Design review of the part shown in the three views and the two pictorial views. Dimensions are in mm from the part's minimum x, y and z. A direction names the side the tool comes from. Coordinates: 2 decimals unless noted, no trailing zeros. Loops run counter-clockwise (first coordinate to the right, second up) from the corner with the lowest first, then second, coordinate; pieces in that order, holes last. Notation, with made-up numbers: (-28.75, 60) -> (-12.75, 60) arc R30 cw to (-12.75, 83) -> close; hole circle Ø9 at (68.25, 35.25). An arc over 180 degrees is marked (long way). Answer in a Markdown table with one row per item.
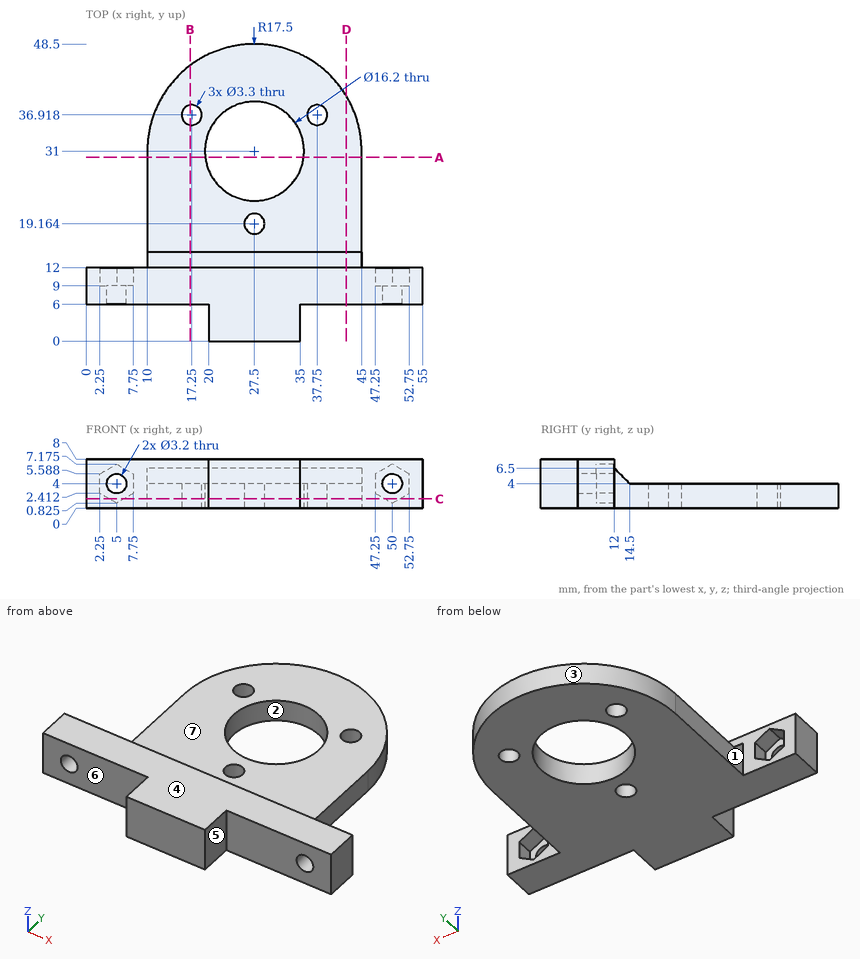
Item 1: For L1, parallel to Z at x = 50, y = 7; L2, parallel to X at y = 10.5, z = 2.25; L3, parallel to Z at x = 14.5, y = 31.5, list the stretches that pass through material, from the lowest coordinate up.
Worked answers:
| item | result |
|---|---|
| L1 | 0 to 2.4, 5.6 to 8 |
| L2 | 0 to 2.53, 7.47 to 47.53, 52.47 to 55 |
| L3 | 0 to 4 |
Item 2: Take a section at A-A, the plane y = 30. State the section outline as (x, z) points.
Worked answers:
| item | result |
|---|---|
| outline | (10, 0) -> (19.46, 0) -> (19.46, 4) -> (10, 4) -> close; (35.54, 0) -> (45, 0) -> (45, 4) -> (35.54, 4) -> close |
Item 3: For the marked faces 4, 5, 6 and 7, list the 3-axis set-ups (+Z, -Z, +X, -X, +Y, -Y) from which the entire face can be reached by the end or side of a thin tool; tool diameter is ignored.
Worked answers:
| item | result |
|---|---|
| face 4 | +Z, +X, -X, +Y, -Y |
| face 5 | +Z, -Z, +X, -Y |
| face 6 | +Z, -Z, -X, -Y |
| face 7 | +Z, +X, -X, +Y |
Item 4: Take a section at D-D, the plane x = 42.5. State the section outline as (y, z) points, and give its area (3 significant figures).
Worked answers:
| item | result |
|---|---|
| outline | (6, 0) -> (40.01, 0) -> (40.01, 4) -> (14.5, 4) -> (12, 6.5) -> (12, 8) -> (6, 8) -> close |
| area | 163 mm² |
Item 5: Take a section at C-C, the plane z = 1.5. Count the separate pieces of the cut face and the enclosed holes in it, and give its area (3 significant figures).
Worked answers:
| item | result |
|---|---|
| separate pieces | 1 |
| enclosed holes | 4 |
| area | 1,320 mm² |
Item 6: The part is to be moulded in two halves that separate along X. For the marked faces 1, 2 and 3, say which applies: +X half, -X half, draft (parallel to the pull), parting line (faces both ways), or undercut.
Worked answers:
| item | result |
|---|---|
| face 1 | -X half |
| face 2 | undercut |
| face 3 | parting line |
Item 7: Insertion check: pin 1 (1.6 mm diameter, centred on x = 49.5, z = 3, fed in from +Y); pin 2 (4 mm diameter, centred on x = 45.5, z = 2.5, fed in from -Y); pin 3 (1 mm diameter, centred on y = 32, z = 1.5, fed in from +X). Each pin has a flat end and moves straight along its axis. Give the tip position at first contact, or say it passes through.
Worked answers:
| item | result |
|---|---|
| pin 1 | y = 9 |
| pin 2 | y = 6 |
| pin 3 | x = 44.99 |
Item 8: Take a section at B-B, the plane x = 17. State the section outline as (y, z) points, and give its area (3 significant figures).
Worked answers:
| item | result |
|---|---|
| outline | (6, 0) -> (35.29, 0) -> (35.29, 4) -> (14.5, 4) -> (12, 6.5) -> (12, 8) -> (6, 8) -> close; (38.55, 0) -> (45, 0) -> (45, 4) -> (38.55, 4) -> close |
| area | 170 mm² |
